Here's how the part is built. I have some questions about the finished solid (model axes, mm). Face numbers are marked on the shaded views. Round coordinates to 2 decimals unless told otherwise and drop trailing zeros. Write each loop counter-clockwise with the first axis right and the second up, starting at its lowest first coordinate (ties: lowest second). Pieces come first, ordered by that corner, then holes. Notation, with made-up numbers: (-18, 39.25) - (38, 39.25) arc R15 ccw to (38, 56.25) - close; hole circle Ø8 at (-23, -8.5). An arc over 180 degrees is marked (long way). One line per question, with ' | ' between items. Start each with the question number.
(1) Imagine slicing it at C-C (x = 8). Write out the boundary of the cut face in (y, z), plus the area to 3 significant figures.
(2) Will these pins go through, and if not, where does the flat tip stop? pin 1 (5 mm diameter, centred on x = 25, z = 16, fed in from +Y); pin 2 (10 mm diameter, centred on y = 17.5, z = 2.5, fed in from -X); pin 3 (5 mm diameter, centred on x = 14, y = 8.5, fed in from -Z); pin 4 (9 mm diameter, centred on y = 0, z = 0, fed in from -X).
(3) Imagine slicing it at A-A (z = 0). Write out the boundary of the cut face in (x, y), plus the area to 3 significant figures.
(4) If I drill on L1, parallel to Z at x = 33.5, y = 0; L2, parallel to X at y = -19, z = -9.5; L3, parallel to X at y = 4, z = 8, over which ranges is the centre line in solid material (lowest first)?
(5) Thinking about a two-plate mould opening in Y: for the marked faces 1, 2 and 3, which applies, pulls with the +Y half, pulls with the -Y half, needs draft (parallel to the pull), parting line crosses it, or undercut?
(6) Imagine slicing it at D-D (z = 16). Write out the boundary of the cut face in (x, y).
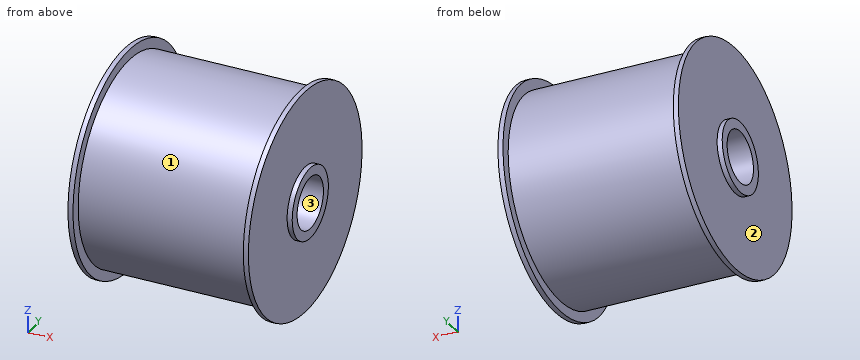
Autodesk Inventor part; units mm, degrees
ref_plane "YZ Plane" through (0, 0, 0) normal (1, 0, 0) x (0, 1, 0)
ref_plane "XZ Plane" through (0, 0, 0) normal (0, 1, 0) x (-1, 0, 0)
ref_plane "XY Plane" through (0, 0, 0) normal (0, 0, 1) x (1, 0, 0)
sketch "スケッチ1" plane through (0, 0, 0) normal (1, 0, 0) x (0, 1, 0)
  circle A0 centre (0, 0) radius 20
  dimension "d0" = 40
extrude "押し出し1" add sketch "スケッチ1" along normal blind 33.6
sketch "スケッチ2" plane through (33.6, 0, 0) normal (1, 0, 0) x (0, 0, -1)
  circle A0 centre (0, 0) radius 22
  dimension "d3" = 44
extrude "押し出し2" add sketch "スケッチ2" along normal blind 1
sketch "スケッチ3" plane through (34.6, 0, 0) normal (1, 0, 0) x (0, 0, -1)
  circle A0 centre (0, 0) radius 7
  dimension "d6" = 14
extrude "押し出し3" add sketch "スケッチ3" along normal blind 1
sketch "スケッチ4" plane through (0, 0, 0) normal (-1, 0, 0) x (0, 0, 1)
  circle A0 centre (0, 0) radius 22
  dimension "d9" = 44
extrude "押し出し4" add sketch "スケッチ4" along normal blind 1
sketch "スケッチ5" plane through (-1, 0, 0) normal (-1, 0, 0) x (0, 0, 1)
  circle A0 centre (0, 0) radius 7
  dimension "d12" = 14
extrude "押し出し5" add sketch "スケッチ5" along normal blind 1
sketch "スケッチ6" plane through (35.6, 0, 0) normal (1, 0, 0) x (0, 0, -1)
  circle A0 centre (0, 0) radius 7
hole "穴1" at (35.6, 0, 0) direction (-1, 0, 0) diameter 10.2 end through all
properties part number "CLS_typeC_31.4N"
Check sheet entries:
1) outline: circle Ø40 at (0, 0); hole circle Ø10.2 at (0, 0) | area: 1,170 mm^2
2) pin 1: y = 14.76 | pin 2: x = -1 | pin 3: z = -19.08 | pin 4: through
3) outline: (-2, -7) - (-1, -7) - (-1, -22) - (0, -22) - (0, -20) - (33.6, -20) - (33.6, -22) - (34.6, -22) - (34.6, -7) - (35.6, -7) - (35.6, -5.1) - (-2, -5.1) - close; (-2, 5.1) - (35.6, 5.1) - (35.6, 7) - (34.6, 7) - (34.6, 22) - (33.6, 22) - (33.6, 20) - (0, 20) - (0, 22) - (-1, 22) - (-1, 7) - (-2, 7) - close | area: 1,080 mm^2
4) L1: -20 to -5.1, 5.1 to 20 | L2: -1 to 0, 33.6 to 34.6 | L3: -1 to 34.6
5) face 1: parting line crosses it | face 2: needs draft | face 3: undercut
6) outline: (-1, -15.1) - (0, -15.1) - (0, -12) - (33.6, -12) - (33.6, -15.1) - (34.6, -15.1) - (34.6, 15.1) - (33.6, 15.1) - (33.6, 12) - (0, 12) - (0, 15.1) - (-1, 15.1) - close
